Source: CAD feature listing. Evaluate the final solid. Frame: model axes, mm. Face numbers are marked on the shaded views. A direction names the side the tool comes from. Coordinates: 2 decimals unless noted, no trailing zeros. Write each loop counter-clockwise with the first axis right and the second up, starting at its lowest first coordinate (ties: lowest second). Pieces come first, ordered by that corner, then holes. Notation, with made-up numbers: (60, 66) - (83, 66) arc R20 cw to (83, 78) - close; hole circle Ø5 at (67.25, 35.5). An arc over 180 degrees is marked (long way). One line per question, with ' | ' between items. Start each with the question number.
Q1. Contact query for flat-ended pins moving along their axis: P1, Ø1, axis at y = 0.5, z = 1, coming from the +X side; P2, Ø9.5, axis at x = 0, z = 0, coming from the -Y side; P3, Ø6, axis at x = 11, y = -1, coming from the -Z side; P4, Ø2.5, axis at x = 8.5, z = -4, coming from the +Y side. Output: stop coordinate, or through.
Q2. Cut plane A-A, the plane z = 0. Return loops of the section in (x, y) (3 decimals).
Q3. Cut plane C-C, the plane y = -4.5. Give the number of separate pieces and of enclosed holes in the cut face, plus the area to 3 significant figures.
Q4. Access query for the marked faces 1, 2, 3 and 4. Directions: +Z, -Z, +X, -X, +Y, -Y. A direction counts if a zero-diameter tool reaches every point of the face in a straight line with its end or side. Return the directions, or none.
Q5. Line query: line 1 (X direction, y = -5.85, z = 0) (3 decimals); line 2 (Y direction, x = 5.25, z = -12.75) (3 decimals); line 3 (Y direction, x = -6.75, z = 5.75) (3 decimals). Output: solid intervals per line, ascending.
Q6. Draft query along X for the marked faces 5, 6 and 7. Return one class per face: +X half, -X half, draft (parallel to the pull), parting line (faces both ways), or undercut.
Q7. Cut plane B-B, the plane x = 0. Return loops of the section in (y, z) (3 decimals).
```python
from build123d import *

# Parameters (mm, degrees)
CUT_EXTRUDE3_REACH             = 24.395
SKETCH6_W                      = 1.27
SKETCH6_H                      = 13.462
CUT_EXTRUDE3_DIRECTION_2_DEPTH = 23.394615982
CIRPATTERN1_COUNT              = 8


with BuildPart() as part:
    # Sketch5 → Revolve1 (revolve)
    with BuildSketch(Plane.XY, mode=Mode.PRIVATE) as revolve1_sk:
        Polygon((-11.249999979, -3.5), (-11.249999979, 3.5), (-11.557, 3.5), (-13.462, 0.602345319), (-12.7, 0.325), (-12.7, -5.775), (-13.97, -5.775), (-13.97, -7.045), (-8.074999979, -7.045), (-8.074999979, -3.5), align=None)
    revolve(revolve1_sk.sketch.rotate(Axis((0, 0.325, 0), (0, -1, 0)), 270), axis=Axis((0, 0.325, 0), (0, -1, 0)))

    # Cut-Extrude3: up to this face of the body (flat: up to its plane)
    cut_extrude3_end = Plane(part.part.faces().sort_by_distance((0, -5.775, -13.095131269))[0])
    # Sketch6 → Cut-Extrude3 (cut, up to the picked face)
    with BuildSketch(Plane(origin=(0, 3.5, 0), x_dir=(1, 0, 0), z_dir=(0, 1, 0)), mode=Mode.PRIVATE) as cut_extrude3_sk1:
        with Locations((0, 6.731)):
            Rectangle(SKETCH6_W, SKETCH6_H)
    cut_extrude3_tool1 = split(extrude(cut_extrude3_sk1.sketch, amount=-CUT_EXTRUDE3_REACH, mode=Mode.PRIVATE), bisect_by=cut_extrude3_end, keep=Keep.BOTH, mode=Mode.PRIVATE)
    cut_extrude3 = cut_extrude3_tool1.solids().sort_by(Axis((0, 3.5, -6.731), (0, -1, 0)))[0]
    add(cut_extrude3, mode=Mode.SUBTRACT)

    # Sketch6 → Cut-Extrude3 direction 2 (cut)
    with BuildSketch(Plane(origin=(0, 3.5, 0), x_dir=(1, 0, 0), z_dir=(0, 1, 0))):
        with Locations((0, 6.731)):
            Rectangle(SKETCH6_W, SKETCH6_H)
    cut_extrude3_direction_2 = extrude(amount=CUT_EXTRUDE3_DIRECTION_2_DEPTH, mode=Mode.SUBTRACT)

    # CirPattern1: Cut-Extrude3, Cut-Extrude3 direction 2 ×8 about axis
    cirpattern1_axis = Axis((0, 0, 0), (0, 1, 0))
    add([cut_extrude3.rotate(cirpattern1_axis, i * 360 / CIRPATTERN1_COUNT) for i in range(1, CIRPATTERN1_COUNT)], mode=Mode.SUBTRACT)
    add([cut_extrude3_direction_2.rotate(cirpattern1_axis, i * 360 / CIRPATTERN1_COUNT) for i in range(1, CIRPATTERN1_COUNT)], mode=Mode.SUBTRACT)


solid = part.part
```
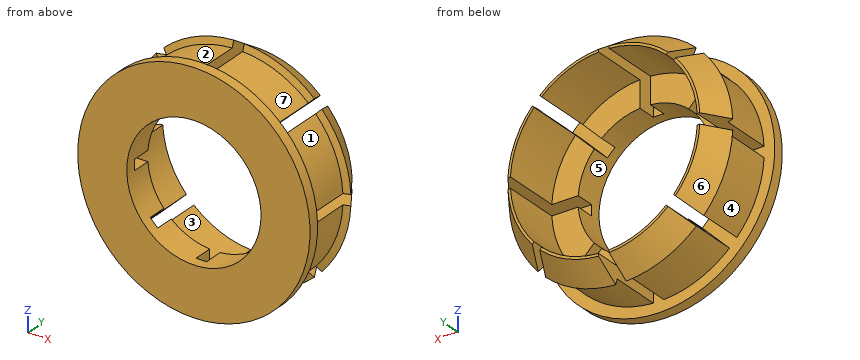
Reply:
1) P1: stops at x = 13.45 | P2: passes through | P3: stops at z = -10.47 | P4: stops at y = -3.5
2) outline: (-13.97, -7.045) - (-8.075, -7.045) - (-8.075, -5.775) - (-13.97, -5.775) - close; (8.075, -7.045) - (13.97, -7.045) - (13.97, -5.775) - (8.075, -5.775) - close
3) separate pieces: 8 | enclosed holes: 0 | area: 255 mm^2
4) face 1: +Z, +X | face 2: +Z, -X | face 3: +Y | face 4: -Z, -X
5) line 1: x = -13.97 to -8.075, 8.075 to 13.97 | line 2: y = -7.045 to -5.775 | line 3: y = -7.045 to -3.5
6) face 5: undercut | face 6: -X half | face 7: +X half
7) outline: (-7.045, -13.97) - (-5.775, -13.97) - (-5.775, -8.075) - (-7.045, -8.075) - close; (-7.045, 8.075) - (-5.775, 8.075) - (-5.775, 13.97) - (-7.045, 13.97) - close
